Model file for the job. Use its own axes, mm. A direction names the side the tool comes from. Give positions to 0.01 mm unless a question says otherwise; leave off trailing zeros. Write each loop counter-clockwise with the first axis right and the second up, starting at its lowest first coordinate (ties: lowest second). Pieces come first, ordered by that corner, then holes. Notation, with made-up numbers: (35, 38.5) - (66, 38.5) arc R33 cw to (66, 72.5) - close; hole circle Ø6 at (-27, -29.5). An arc over 180 degrees is marked (long way). One line per item, written item: value. Start each with the question number.
(1) Cut at A-A, the plane z = -31. List the corners of the cut face in (x, y), and give its area (3 significant figures).
(2) Probe L1, parallel to Y at x = 40.5, z = -9.5; L2, parallel to Z at x = 22, y = -68.25; L3, parallel to X at y = -71, z = -15.5. List the from-to ranges inside material, lowest first.
(3) Drop flat-ended pins along their axis: P1, Ø7.5, axis at x = 4, z = -12, coming from the +Y side; P2, Ø8, axis at y = -66, z = -7, coming from the -X side; P3, Ø12, axis at x = 14, y = -59, coming from the -Z side. Give the stop position or say it passes through.
(4) 3-axis set-ups, long thin cutter, end or side, ignore diameter. For faces 4 (the face through (22, -66, -19)), 5 (the face through (22, -51, -12)): which of +Z, -Z, +X, -X, +Y, -Y reach the whole face in a straight line?
(5) Cut at B-B, the plane z = -1. List the corners of the cut face in (x, y).
(6) Mould opens along X. For faces 1 (the face through (-2.195, -72.549, -11.282)), 2 (the face through (22, -69, -29)), 3 (the face through (16.1, -58.61, -10.05)) say: pulls with the +X half, pulls with the -X half, needs draft (parallel to the pull), parting line crosses it, or undercut.
from build123d import *

# Parameters (mm, degrees)
CYLINDER011_R             = 8
CYLINDER011_DEPTH         = 7
CYLINDER012_R             = 8
CYLINDER012_DEPTH         = 7
CYLINDER010_R             = 8
CYLINDER010_DEPTH         = 7
CYLINDER009_R             = 8
CYLINDER009_DEPTH         = 7
CYLINDER005_R             = 6.5
CYLINDER005_DEPTH         = 25
CYLINDER006_R             = 10
CYLINDER006_DEPTH         = 10
FUSION001_ROLL_ANGLE      = 90
FUSION001_PITCH_ANGLE     = -7e-06
FUSION001_PLACEMENT_ANGLE = -179.999993


with BuildPart() as cylinder011:
    # Cylinder011 → Cylinder011 (new body)
    with BuildSketch(Plane(origin=(16.4955, 0.685902, 0), x_dir=(1, 0, 0), z_dir=(0, 0, 1))):
        Circle(CYLINDER011_R)
    extrude(amount=CYLINDER011_DEPTH)


with BuildPart() as cylinder012:
    # Cylinder012 → Cylinder012 (new body)
    with BuildSketch(Plane(origin=(-16.3838, -1.44516, 0), x_dir=(1, 0, 0), z_dir=(0, 0, 1))):
        Circle(CYLINDER012_R)
    extrude(amount=CYLINDER012_DEPTH)


with BuildPart() as cylinder010:
    # Cylinder010 → Cylinder010 (new body)
    with BuildSketch(Plane(origin=(0.664718, -16.3626, 0), x_dir=(1, 0, 0), z_dir=(0, 0, 1))):
        Circle(CYLINDER010_R)
    extrude(amount=CYLINDER010_DEPTH)


with BuildPart() as cylinder009:
    # Cylinder009 → Cylinder009 (new body)
    with BuildSketch(Plane(origin=(-0.248596, 16.2122, 0), x_dir=(1, 0, 0), z_dir=(0, 0, 1))):
        Circle(CYLINDER009_R)
    extrude(amount=CYLINDER009_DEPTH)


with BuildPart() as cylinder005:
    # Cylinder005 → Cylinder005 (new body)
    with BuildSketch(Plane.XY):
        Circle(CYLINDER005_R)
    extrude(amount=CYLINDER005_DEPTH)


with BuildPart() as fusion001:
    # Cylinder006 → Cylinder006 (new body)
    with BuildSketch(Plane.XY):
        Circle(CYLINDER006_R)
    extrude(amount=CYLINDER006_DEPTH)

    # Fusion001: union Cylinder011, Cylinder012, Cylinder010, Cylinder009, Cylinder005
    add(cylinder011.part)
    add(cylinder012.part)
    add(cylinder010.part)
    add(cylinder009.part)
    add(cylinder005.part)


with BuildPart() as fusion001_1:
    # Fusion001 roll: moved
    add(fusion001.part.rotate(Axis((0, 0, 0), (1, 0, 0)), FUSION001_ROLL_ANGLE))


with BuildPart() as fusion001_2:
    # Fusion001 pitch: moved
    add(fusion001_1.part.rotate(Axis((0, 0, 0), (0, 1, 0)), FUSION001_PITCH_ANGLE))


with BuildPart() as fusion001_3:
    # Fusion001 placement: moved
    add(fusion001_2.part.moved(Location((22.3, -76, -12))).rotate(Axis((22.3, -76, -12), (0, 0, 1)), FUSION001_PLACEMENT_ANGLE))


solid = fusion001_3.part
Answers follow:
1. outline: (14.08, -76) - (29.19, -76) - (29.19, -69) - (14.08, -69) - close
1. area: 106 mm²
2. L1: y = -76 to -69
2. L2: z = -22 to -2
2. L3: x = -1.01 to 12.62, 12.93 to 46.42
3. P1: stops at y = -69
3. P2: stops at x = -2.02
3. P3: stops at z = -18.08
4. face 4: +Y
4. face 5: +Z, -Z, +X, -X, +Y
5. outline: (16.48, -76) - (28.62, -76) - (28.62, -69) - (16.48, -69) - close
6. face 1: undercut
6. face 2: needs draft
6. face 3: parting line crosses it
